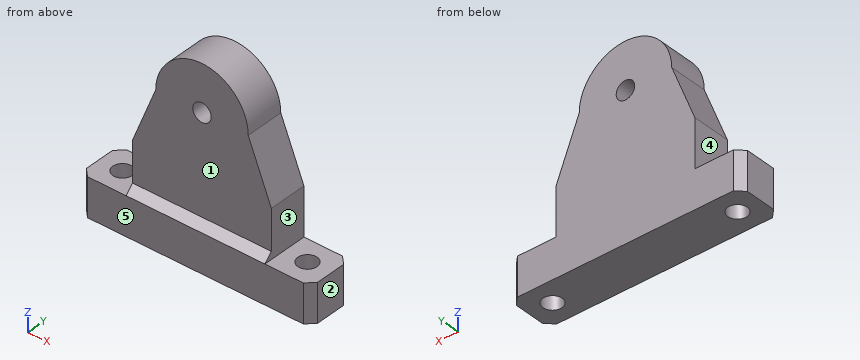
Solid Edge part; units mm, degrees
sketch "Sketch1" plane through (0, 0, 0) normal (0, -1, 0) x (1, 0, 0)
  line L0 (-30, 0) -> (30, 0)
  line L1 (30, 0) -> (30, 10)
  line L2 (30, 10) -> (18, 10)
  line L3 (18, 10) -> (18, 22.5)
  line L4 (18, 22.5) -> (12, 37.5)
  arc A0 (-12, 37.5) -> (12, 37.5) centre (0, 37.5) cw
  line L5 (-18, 22.5) -> (-12, 37.5)
  line L6 (-18, 10) -> (-18, 22.5)
  line L7 (-30, 10) -> (-18, 10)
  line L8 (-30, 0) -> (-30, 10)
  dimension "D1" = 30
  dimension "D2" = 30
  dimension "D3" = 30
  dimension "D4" = 18
  dimension "D5" = 18
extrude "Protrusion1" add sketch "Sketch1" along normal mid plane 12
hole "Hole_1" at (-24, 0, 10) direction (0, 0, -1) diameter 5 end up to next
hole "Hole1" at (24, 0, 10) direction (0, 0, -1) diameter 5 end up to next
sketch "Sketch2" plane through (0, -6, 21.25) normal (0, -1, 0) x (1, 0, 0)
  line L0 (-18, -11.25) -> (18, -11.25)
  line L1 (18, -11.25) -> (18, 28.25)
  line L2 (18, 28.25) -> (-18, 28.25)
  line L3 (-18, 28.25) -> (-18, -11.25)
extrude "ExtrudedCutout_1" cut sketch "Sketch2" against normal blind 2
chamfer "Chamfer_1" distance 2 angle 45 1 edges at (0, -4, 10)
chamfer "Chamfer_2" distance 2 angle 45 4 edges at (30, -6, 5) (30, 6, 5) (-30, -6, 5) (-30, 6, 5)
hole "Hole_3" at (0, -4, 37.5) direction (0, 1, 0) diameter 4.8 end up to next
properties material "Polyethylene, low density"
Verification items for the finished model (mm, model axes). Face numbers are marked on the shaded views. A direction names the side the tool comes from. Give positions to 0.01 mm unless a question says otherwise; leave off trailing zeros. Order: outer loops, then holes, each group sorted by start corner. A loop starts at its lowest first (then second) coordinate and runs counter-clockwise, first axis right, second up. Notation, with made-up numbers: M 86,18 L 106,18 A19 ccw 106,53 Z; hole C -12.75,-30 d1. An arc over 180 degrees is marked long. Return JSON: item names as keys, results as strings. Group by question number.
1) Access from +Z, -Z, +X, -X, +Y, -Y to the whole of each face (thin tool, end or side, straight path). Record for the marked faces 1, 2, 3, 4 and 5.
2) Section check C-C on x = -24. Record the cut outline in (y, z), and give its area (3 significant figures).
3) Scan lines: line 1 (X direction, y = 0, z = 3.5); line 2 (Z direction, x = 0, y = 3.25); line 3 (Y direction, x = -24, z = 5). Record each from-to range of solid material in increasing order.
4) Section check D-D on z = 32. Record the cut outline in (x, y), and give its area (3 significant figures).
5) Section check A-A on y = 0. Record the cut outline in (x, z), and give its area (3 significant figures).
6) Go/stop test with flat-tipped pins: pin 1 Ø4.5 at (x, z) = (0, 37.5) entering from -Y; pin 2 Ø1 at (y, z) = (0.5, 12.5) entering from +X; pin 3 Ø6 at (x, y) = (-6.5, -1.5) entering from +Z; pin 4 Ø11 at (x, z) = (7, 22) entering from -Y. Record where each tip stops, or that it passes through.
Answer block:
{
 "1": {"face 1": "+Z, +X, -X, -Y", "face 2": "+Z, -Z, +X, +Y, -Y", "face 3": "+Z, +X, +Y, -Y", "face 4": "+Z, -X, +Y, -Y", "face 5": "+Z, -Z, +X, -X, -Y"},
 "2": {"outline": "M -6,0 L -2.5,0 L -2.5,10 L -6,10 Z; M 2.5,0 L 6,0 L 6,10 L 2.5,10 Z", "area": "70.0 mm^2"},
 "3": {"line 1": "x = -30 to -26.5, -21.5 to 21.5, 26.5 to 30", "line 2": "z = 0 to 35.1, 39.9 to 49.5", "line 3": "y = -6 to -2.5, 2.5 to 6"},
 "4": {"outline": "M -14.2,-4 L 14.2,-4 L 14.2,6 L -14.2,6 Z", "area": "284 mm^2"},
 "5": {"outline": "M -30,0 L -26.5,0 L -26.5,10 L -30,10 Z; M -21.5,0 L 21.5,0 L 21.5,10 L 18,10 L 18,22.5 L 12,37.5 A12 ccw -12,37.5 L -18,22.5 L -18,10 L -21.5,10 Z; M 26.5,0 L 30,0 L 30,10 L 26.5,10 Z; hole C 0,37.5 d4.8", "area": "1,610 mm^2"},
 "6": {"pin 1": "passes through", "pin 2": "stops at x = 18", "pin 3": "stops at z = 48.98", "pin 4": "stops at y = -4"}
}
